Can you work these out from the drawing? Everything is in mm from the part's minimum corner. A direction names the side the tool comes from. Round coordinates to 2 decimals unless told otherwise and drop trailing zeros. Order: outer loops, then holes, each group sorted by start corner. A loop starts at its lowest first (then second) coordinate and runs counter-clockwise, first axis right, second up. Notation, with made-up numbers: (44, -27.5) - (64, -27.5) arc R16 ccw to (64, -19.5) - close; hole circle Ø10 at (-4, -13). An arc over 180 degrees is marked (long way). Write item = value, one per line.
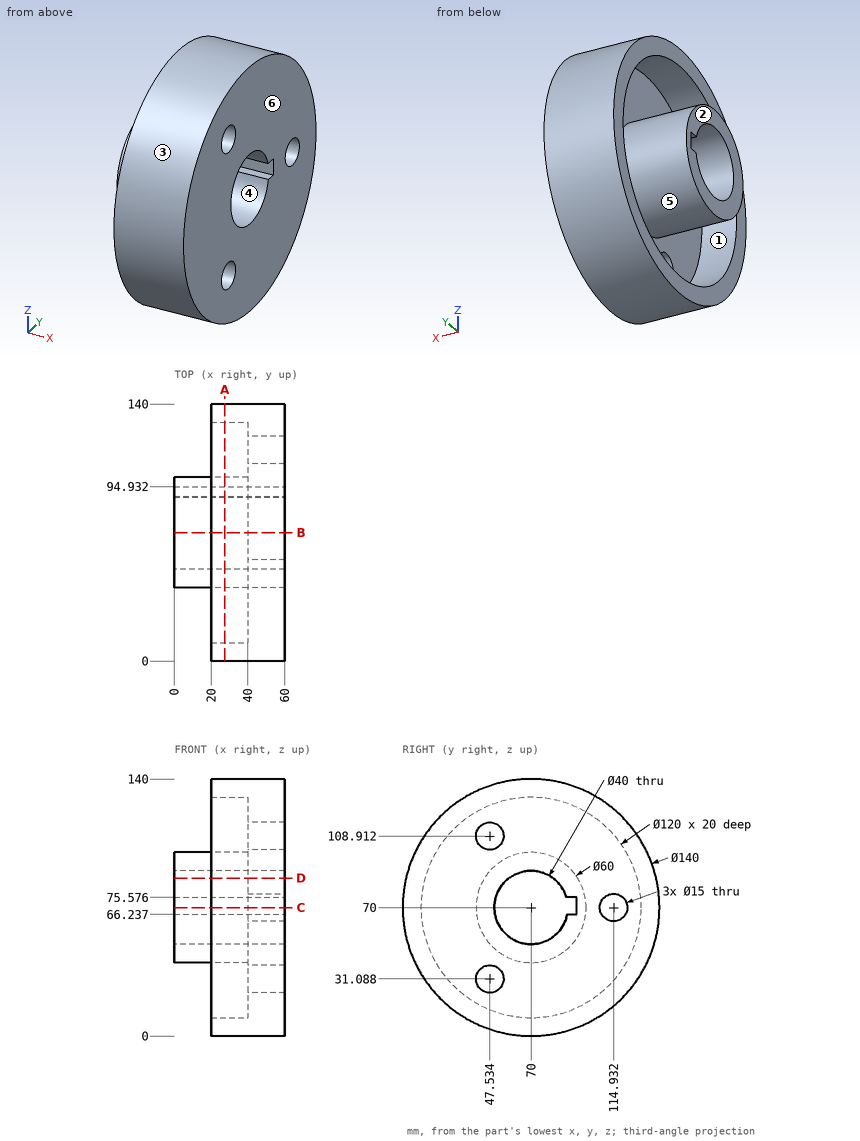
(1) If we section it at C-C (z = 70): Write out the boundary of the cut face in (x, y).
Computed:
outline = (0, 40) - (40, 40) - (40, 10) - (20, 10) - (20, 0) - (60, 0) - (60, 50) - (0, 50) - close; (0, 94.93) - (60, 94.93) - (60, 107.43) - (40, 107.43) - (40, 100) - (0, 100) - close; (20, 130) - (40, 130) - (40, 122.43) - (60, 122.43) - (60, 140) - (20, 140) - close
(2) Will these pins go through, and if not, where does the flat tip stop? P1, Ø4, axis at x = 34, y = 107, coming from the +Z side; P2, Ø2, axis at x = 13.5, z = 93.5, coming from the -Y side; P3, Ø1, axis at x = 23.5, z = 20.5, coming from the -Y side; P4, Ø3, axis at x = 25, z = 71.5, coming from the -Y side.
Computed:
P1 = 130.62
P2 = 50.16
P3 = 20.01
P4 = 0
(3) If we section it at D-D (z = 86): Write out the boundary of the cut face in (x, y).
Computed:
outline = (0, 44.62) - (40, 44.62) - (40, 12.17) - (20, 12.17) - (20, 1.85) - (60, 1.85) - (60, 58) - (0, 58) - close; (0, 82) - (60, 82) - (60, 138.15) - (20, 138.15) - (20, 127.83) - (40, 127.83) - (40, 95.38) - (0, 95.38) - close
(4) If I drill on line 1 (Z direction, x = 27.5, y = 70); line 2 (Y direction, x = 45, z = 66) (1 decimal); line 3 (Z direction, x = 32, y = 66) (1 decimal), over which ranges is the centre line in solid material (lowest first)? Write a range as from..to.
Computed:
line_1 = 0..10, 40..50, 90..100, 130..140
line_2 = 0.1..50.4, 89.6..108.6, 121.3..139.9
line_3 = 0.1..10.1, 40.3..50.4, 89.6..99.7, 129.9..139.9
(5) On a 3-axis mill with a long thin cutter (end or side, diameter ignored), from which of +Z, -Z, +X, -X, +Y, -Y can I reach the whole of each face in a straight line? I mean the marked faces 5 and 6. Say none if no direction works.
Computed:
face_5 = -X
face_6 = +Z, -Z, +X, +Y, -Y
(6) Thinking about a two-plate mould opening in Y: for the marked faces 1, 2, 3 and 4, which applies, +Y half, -Y half, draft (parallel to the pull), parting line (faces both ways), or undercut?
Computed:
face_1 = undercut
face_2 = draft
face_3 = parting line
face_4 = undercut
(7) If we section it at A-A (x = 27.5): Write out the boundary of the cut face in (y, z) (1 decimal).
Computed:
outline = circle Ø140 at (70, 70); circle Ø60 at (70, 70); hole circle Ø120 at (70, 70); hole (89.2, 75.6) arc R20 ccw (long way) to (89.6, 66.2) - (94.9, 66.2) - (94.9, 75.6) - close
(8) If we section it at B-B (y = 70): Write out the boundary of the cut face in (x, z).
Computed:
outline = (0, 40) - (40, 40) - (40, 10) - (20, 10) - (20, 0) - (60, 0) - (60, 50) - (0, 50) - close; (0, 90) - (60, 90) - (60, 140) - (20, 140) - (20, 130) - (40, 130) - (40, 100) - (0, 100) - close
